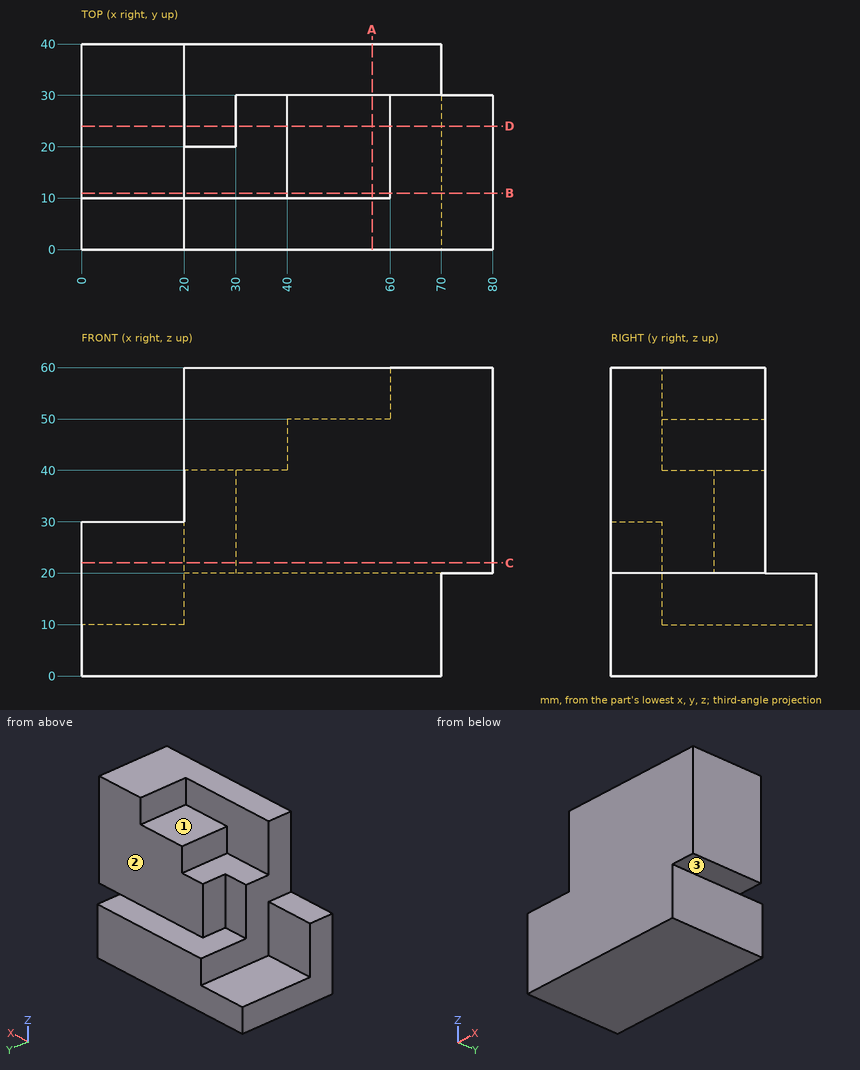
Input: dimensioned drawing with shaded views. Units: mm. Origin: part minimum x, y, z. A direction names the side the tool comes from. Round coordinates to 2 decimals unless told otherwise and drop trailing zeros. Order: outer loops, then holes, each group sorted by start corner. A loop starts at its lowest first (then second) coordinate and runs counter-clockwise, first axis right, second up. Notation, with made-up numbers: (71.5, 77.25) -> (83.5, 77.25) arc R23 cw to (83.5, 86.25) -> close; hole circle Ø1 at (48.25, -15). An arc over 180 degrees is marked (long way). One line per item, written item: value. Start each with the question number.
Q1. Pin query (flat end, axial travel): pin 1 (20 mm diameter, centred on x = 43.5, z = 44.5, fed in from +Y); pin 2 (16 mm diameter, centred on x = 50, y = 17.5, fed in from +Z); pin 3 (6 mm diameter, centred on x = 56.5, y = 32.5, fed in from +Z); pin 4 (6 mm diameter, centred on x = 14, z = 16, fed in from +Y). Return the tip coordinate at first contact, or that it passes through.
Q2. Material intervals for probe 1 along Y at (x, z) = (31, 50.5); probe 2 along X at (y, z) = (24, 49); probe 3 along Z at (x, y) = (72, 15), sorted ascending.
Q3. Section query A-A (x = 56.5). Return the cut outline in (y, z), plus the area to 3 significant figures.
Q4. Access query for the marked faces 1, 2 and 3. Directions: +Z, -Z, +X, -X, +Y, -Y. A direction counts if a zero-diameter tool reaches every point of the face in a straight line with its end or side. Return the directions, or none.
Q5. Section query B-B (y = 11). Return the cut outline in (x, z).
Q6. Section query D-D (y = 24). Return the cut outline in (x, z), plus the area to 3 significant figures.
Q7. Section query C-C (z = 22). Return the cut outline in (x, y), plus the area to 3 significant figures.
Findings below:
1. pin 1: y = 30
1. pin 2: z = 60
1. pin 3: z = 50
1. pin 4: y = 10
2. probe 1: 0 to 10
2. probe 2: 40 to 80
2. probe 3: 20 to 60
3. outline: (0, 0) -> (40, 0) -> (40, 20) -> (30, 20) -> (30, 50) -> (10, 50) -> (10, 60) -> (0, 60) -> close
3. area: 1,800 mm²
4. face 1: +Z, -X, +Y
4. face 2: +Z, +X, -X, +Y
4. face 3: -Z, +X, +Y, -Y
5. outline: (0, 0) -> (70, 0) -> (70, 20) -> (80, 20) -> (80, 60) -> (60, 60) -> (60, 50) -> (40, 50) -> (40, 40) -> (20, 40) -> (20, 10) -> (0, 10) -> close
6. outline: (0, 0) -> (70, 0) -> (70, 20) -> (80, 20) -> (80, 60) -> (60, 60) -> (60, 50) -> (40, 50) -> (40, 40) -> (30, 40) -> (30, 20) -> (20, 20) -> (20, 10) -> (0, 10) -> close
6. area: 2,800 mm²
7. outline: (0, 0) -> (80, 0) -> (80, 30) -> (30, 30) -> (30, 20) -> (20, 20) -> (20, 10) -> (0, 10) -> close
7. area: 1,900 mm²
